Design review of the part built by this model. Coordinates are the model's own, in mm. A direction names the side the tool comes from. Coordinates: 2 decimals unless noted, no trailing zeros. Write each loop counter-clockwise with the first axis right and the second up, starting at its lowest first coordinate (ties: lowest second). Pieces come first, ordered by that corner, then holes. Notation, with made-up numbers: (-37, 37) - (2, 37) arc R29 cw to (2, 57) - close; hole circle Ø7 at (-6, -31.75). An arc over 180 degrees is marked (long way). Use a Markdown table: item, result.
from build123d import *

# Parameters (mm, degrees)
SKETCH1_W                                           = 101.6
SKETCH1_H                                           = 101.6
BOSS_EXTRUDE1_DEPTH                                 = 3.81
M6X1_0_TAPPED_HOLE1_D                               = 5
M6X1_0_TAPPED_HOLE1_DEPTH                           = 14.986
M6X1_0_TAPPED_HOLE1_TIP                             = 1.502151548
SKETCH4_W                                           = 101.6
SKETCH4_H                                           = 67.31
BOSS_EXTRUDE2_DEPTH                                 = 5.715
SKETCH7_W                                           = 101.6
SKETCH7_H                                           = 9.525
BOSS_EXTRUDE3_DEPTH                                 = 32.385
DZ_START                                            = -5.715
DZ_SLOT_DEPTH                                       = 9.525
RIB_1_BOSS_EXTRUDE4_DEPTH                           = 9.525
RIB_2_BOSS_EXTRUDE5_DEPTH                           = 9.525
CSK_FOR_1_4_FLAT_HEAD_SOCKET_CAP_SCREW1_D           = 6.7564
CSK_FOR_1_4_FLAT_HEAD_SOCKET_CAP_SCREW1_CSINK_D     = 13.4874
CSK_FOR_1_4_FLAT_HEAD_SOCKET_CAP_SCREW1_CSINK_ANGLE = 82


# Read off the part's stored shape, not the designer's step: dz slot
with BuildPart() as part:
    # Sketch1 → Boss-Extrude1 (new body)
    with BuildSketch(Plane.XY):
        with Locations((-50.8, 88.9)):
            Rectangle(SKETCH1_W, SKETCH1_H)
    extrude(amount=BOSS_EXTRUDE1_DEPTH)

    # M6x1.0 Tapped Hole1
    with Locations(Plane(origin=(-50.8, 0, 0), x_dir=(-1, 0, 0), z_dir=(0, 0, -1))):
        with Locations((-30.795161674, 53.586240129), (29.387245779, 53.586240129)):
            Hole(M6X1_0_TAPPED_HOLE1_D / 2, depth=M6X1_0_TAPPED_HOLE1_DEPTH)
            with Locations((0, 0, -(M6X1_0_TAPPED_HOLE1_DEPTH + M6X1_0_TAPPED_HOLE1_TIP / 2))):  # 118° drill point
                Cone(0, M6X1_0_TAPPED_HOLE1_D / 2, M6X1_0_TAPPED_HOLE1_TIP, mode=Mode.SUBTRACT)

    # Sketch4 → Boss-Extrude2 (add)
    with BuildSketch(Plane(origin=(0, 0, 0), x_dir=(-1, 0, 0), z_dir=(0, 0, -1))):
        with Locations((50.8, 106.045)):
            Rectangle(SKETCH4_W, SKETCH4_H)
    extrude(amount=BOSS_EXTRUDE2_DEPTH)

    # Sketch7 → Boss-Extrude3 (add)
    with BuildSketch(Plane(origin=(0, 0, -5.715), x_dir=(-1, 0, 0), z_dir=(0, 0, -1))):
        with Locations((50.8, 77.1525)):
            Rectangle(SKETCH7_W, SKETCH7_H)
    extrude(amount=BOSS_EXTRUDE3_DEPTH)

    # dz slot outline → dz slot (cut)
    with BuildSketch(Plane.XY.offset(DZ_START)):
        with BuildLine():
            ThreePointArc((-47.4218, 129.5146), (-50.8, 132.8928), (-54.1782, 129.5146))
            Line((-54.1782, 129.5146), (-54.1782, 91.6432))
            ThreePointArc((-54.1782, 91.6432), (-50.8, 88.265), (-47.4218, 91.6432))
            Line((-47.4218, 91.6432), (-47.4218, 129.5146))
        make_face()
    extrude(amount=DZ_SLOT_DEPTH, mode=Mode.SUBTRACT)

    # rib 1 Sketch9 → rib 1 Boss-Extrude4 (add)
    with BuildSketch(Plane(origin=(0, 0, 0), x_dir=(0, 0, -1), z_dir=(1, 0, 0))):
        Polygon((38.1, 81.915), (38.1, 88.265), (12.065, 139.7), (5.715, 139.7), (5.715, 81.915), align=None)
    extrude(amount=-RIB_1_BOSS_EXTRUDE4_DEPTH)

    # Sketch10 → rib 2 Boss-Extrude5 (add)
    with BuildSketch(Plane.ZY.offset(101.6)):
        Polygon((-38.1, 81.915), (-5.715, 81.915), (-5.715, 139.7), (-12.065, 139.7), (-38.1, 88.265), align=None)
    extrude(amount=-RIB_2_BOSS_EXTRUDE5_DEPTH)

    # CSK for 1/4 Flat Head Socket Cap Screw1 (through all)
    with Locations(Plane(origin=(-50.8, 81.915, -38.1), x_dir=(1, 0, 0), z_dir=(0, 1, 0))):
        with Locations((19.05, -19.05), (-19.05, -19.05)):
            CounterSinkHole(CSK_FOR_1_4_FLAT_HEAD_SOCKET_CAP_SCREW1_D / 2, CSK_FOR_1_4_FLAT_HEAD_SOCKET_CAP_SCREW1_CSINK_D / 2, counter_sink_angle=CSK_FOR_1_4_FLAT_HEAD_SOCKET_CAP_SCREW1_CSINK_ANGLE)


solid = part.part
(1) For pin 1 (3 mm diameter, centred on x = -84, z = -17.5, fed in from -Y); pin 2 (8 mm diameter, centred on x = -20, y = 53.59, fed in from -Z); pin 3 (9.5 mm diameter, centred on x = -39.5, z = -16, fed in from +Y) (3 decimals), all flat-tipped, find the tip position at first contact; note any pin that passes through.
Determined:
| item | result |
|---|---|
| pin 1 | y = 72.39 |
| pin 2 | z = 0 |
| pin 3 | y = 81.915 |
(2) Take a section at B-B on z = -2. Write out the cut boundary in (x, y), and give its area (3 significant figures).
Determined:
| item | result |
|---|---|
| outline | (-101.6, 72.39) - (0, 72.39) - (0, 139.7) - (-101.6, 139.7) - close; hole (-54.18, 91.64) arc R3.38 ccw to (-47.42, 91.64) - (-47.42, 129.51) arc R3.38 ccw to (-54.18, 129.51) - close |
| area | 6,550 mm2 |
(3) Take a section at C-C on y = 97. Write out the cut boundary in (x, z) (3 decimals).
Determined:
| item | result |
|---|---|
| outline | (-101.6, -33.679) - (-92.075, -33.679) - (-92.075, -5.715) - (-54.178, -5.715) - (-54.178, 3.81) - (-101.6, 3.81) - close; (-47.422, -5.715) - (-9.525, -5.715) - (-9.525, -33.679) - (0, -33.679) - (0, 3.81) - (-47.422, 3.81) - close |
(4) Draft analysis for pull direction Y (two halves, no side actions). For faces 1 (the flat face through (-52, 139.7, -2)), 2 (the flat face through (-52, 79, -38.1)), 3 (the flat face through (-54.178, 111, -1)), 4 (the cylindrical face through (-50.874, 88.266, -1.019)), state which applies: +Y half, -Y half, draft (parallel to the pull), parting line (faces both ways), or undercut.
Determined:
| item | result |
|---|---|
| face 1 | +Y half |
| face 2 | draft |
| face 3 | undercut |
| face 4 | undercut |
(5) Machinability: for faces 5 (the flat face through (-41, 111, -5.715)), 6 (the flat face through (-47.422, 110, -1)), 7 (the flat face through (-52, 55, 0)), 8 (the flat face through (-52, 38.1, 2)), which of the approach directions +Z, -Z, +X, -X, +Y, -Y give a long, thin tool a straight path to every point of the face, cutting with its end or side? Answer none if there is none.
Determined:
| item | result |
|---|---|
| face 5 | -Z, +Y |
| face 6 | +Z, -Z |
| face 7 | -Z, +X, -X, -Y |
| face 8 | +Z, -Z, +X, -X, -Y |
(6) Take a section at D-D on y = 86. Write out the cut boundary in (x, z) (3 decimals).
Determined:
| item | result |
|---|---|
| outline | (-101.6, -38.1) - (-92.075, -38.1) - (-92.075, -5.715) - (-9.525, -5.715) - (-9.525, -38.1) - (0, -38.1) - (0, 3.81) - (-101.6, 3.81) - close |
(7) For L1, parallel to X at y = 76, z = -19; L2, parallel to X at y = 110, z = -20 (3 decimals); L3, parallel to X at y = 109, z = -2, list the stretches that pass through material, from the lowest coordinate up. Write a range as from..to.
Determined:
| item | result |
|---|---|
| L1 | -101.6..-73.23, -66.47..-35.13, -28.37..0 |
| L2 | -101.6..-92.075, -9.525..0 |
| L3 | -101.6..-54.18, -47.42..0 |
(8) Take a section at A-A on x = -50.8. Write out the cut boundary in (y, z) (3 decimals).
Determined:
| item | result |
|---|---|
| outline | (38.1, 0) - (72.39, 0) - (72.39, -38.1) - (81.915, -38.1) - (81.915, -5.715) - (88.265, -5.715) - (88.265, 3.81) - (38.1, 3.81) - close; (132.893, -5.715) - (139.7, -5.715) - (139.7, 3.81) - (132.893, 3.81) - close |
